from build123d import *

# Parameters (mm, degrees)
SKETCH3_W           = 31.27
SKETCH3_H           = 42.48
BOSS_EXTRUDE1_DEPTH = 6
SKETCH4_R           = 4.7
BOSS_EXTRUDE2_DEPTH = 6
SKETCH6_R           = 5.1
CUT_EXTRUDE2_DEPTH  = 6
FILLET1_R           = 2
FILLET2_R           = 2


with BuildPart() as part:
    # Sketch3 → Boss-Extrude1 (new body)
    with BuildSketch(Plane(origin=(0, 0, 0), x_dir=(1, 0, 0), z_dir=(0, 1, 0))):
        Rectangle(SKETCH3_W, SKETCH3_H)
    extrude(amount=BOSS_EXTRUDE1_DEPTH)

    # Sketch4 → Boss-Extrude2 (add)
    with BuildSketch(Plane(origin=(15.635, 0, 0), x_dir=(0, 0, -1), z_dir=(1, 0, 0))):
        with BuildLine():
            Line((-24.997886253, 0), (25.03656642, 0))
            Line((25.03656642, 0), (25.03656642, 10.942584388))
            Line((25.03656642, 10.942584388), (37.020669589, 23))
            Line((37.020669589, 23), (19.258864986, 40.653807887))
            ThreePointArc((19.258864986, 40.653807887), (-11.905269618, 62.875361443), (-15.817481327, 24.800496669))
            Line((-15.817481327, 24.800496669), (-24.997886253, 12.19))
            Line((-24.997886253, 12.19), (-24.997886253, 0))
        make_face()
        with Locations((-2.786694922, 42.7)):
            Circle(SKETCH4_R, mode=Mode.SUBTRACT)
    boss_extrude2 = extrude(amount=BOSS_EXTRUDE2_DEPTH)

    # Mirror2: Boss-Extrude2 across plane
    add(boss_extrude2.mirror(Plane(origin=(0, 0, 0), x_dir=(0, 0, 1), z_dir=(1, 0, 0))))

    # Sketch6 → Cut-Extrude2 (cut)
    with BuildSketch(Plane.XZ):
        with Locations(Location((0, 0, 0), (0, 0, 270))):
            Circle(SKETCH6_R)
    extrude(amount=-CUT_EXTRUDE2_DEPTH, mode=Mode.SUBTRACT)

    # Fillet1
    fillet1_edges = [part.edges().sort_by_distance(p)[0] for p in [
        (-18.635, 12.19, 24.997886253),
        (-18.635, 0, 24.997886253),
        (18.635, 10.942584388, -25.03656642),
        (-18.635, 10.942584388, -25.03656642),
        (-18.635, 0, -25.03656642),
        (18.635, 0, -25.03656642),
        (18.635, 0, 24.997886253),
        (18.635, 12.19, 24.997886253),
        (18.635, 24.800496669, 15.817481327),
        (-18.635, 24.800496669, 15.817481327),
        (18.635, 23, -37.020669589),
        (-18.635, 23, -37.020669589),
    ]]
    fillet(fillet1_edges, radius=FILLET1_R)

    # Fillet2
    fillet2_edges = [part.edges().sort_by_distance(p)[0] for p in [
        (18.635, 40.653807887, -19.258864986),
        (-18.635, 40.653807887, -19.258864986),
    ]]
    fillet(fillet2_edges, radius=FILLET2_R)


solid = part.part
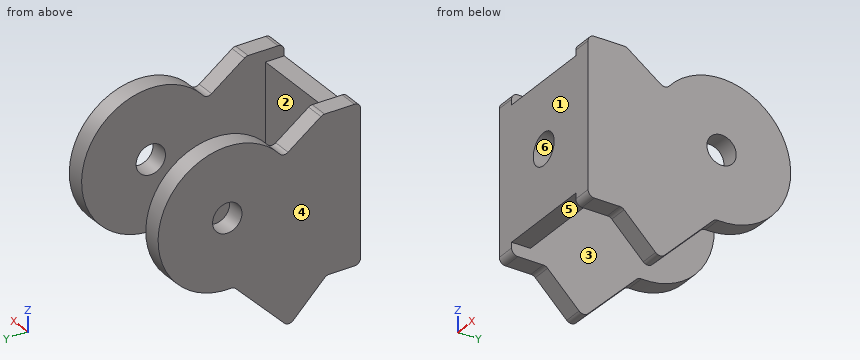
Read the model definition and answer for the solid it produces. Units are mm, in the model's axes. Face numbers are marked on the shaded views. A direction names the side the tool comes from. Round coordinates to 2 decimals unless told otherwise and drop trailing zeros. Write each loop counter-clockwise with the first axis right and the second up, starting at its lowest first coordinate (ties: lowest second). Pieces come first, ordered by that corner, then holes.
1. Straight lines are drawn through the part: L1, parallel to X at y = 3.05, z = 0 (3 decimals); L2, parallel to X at y = 40, z = 22 (3 decimals); L3, parallel to Y at x = -1, z = 5.5. For each, find the intervals that lie inside material, in ascending order.
2. The part is cut by section D-D, the plane z = 6.5. Determine the outline of the cut face in (x, y) (3 decimals), then the cut area to 3 significant figures.
3. Which of the six approach directions +Z, -Z, +X, -X, +Y, -Y give full straight-line access (tool end or side, diameter ignored) to the marked faces 5 and 6?
4. The part is cut by section C-C, the plane y = 7.5. Determine the outline of the cut face in (x, z) (3 decimals), then the cut area to 3 significant figures.
5. The part is cut by section A-A, the plane y = 42.7. Determine the outline of the cut face in (x, z) (3 decimals), then the cut area to 3 significant figures.
6. The part is cut by section B-B, the plane x = 0. Determine the outline of the cut face in (y, z).
7. Given pin 1 Ø10 at (x, z) = (-7, -0.5) entering from +Y; pin 2 Ø6.5 at (x, y) = (18.5, 5) entering from -Z; pin 3 Ø1.8 at (x, y) = (-4, 2.5) entering from +Z; pin 4 Ø3 at (x, y) = (13.5, 46.5) entering from +Z (3 decimals), each flat-ended and moving along its own axis, determine where each tip first touches the part or whether it passes through.
8. Determine the mould class of the marked faces 1, 2, 3 and 4 for opening direction X: pulls with the +X half, pulls with the -X half, needs draft (parallel to the pull), parting line crosses it, or undercut.
Values:
1. L1: x = -21.635 to -5.1, 5.1 to 21.635
1. L2: x = -21.635 to -15.635, 15.635 to 21.635
1. L3: y = 0 to 6
2. outline: (-21.635, 0) - (21.635, 0) - (21.635, 39.819) - (15.635, 39.819) - (15.635, 6) - (-15.635, 6) - (-15.635, 39.819) - (-21.635, 39.819) - close; (-21.635, 45.581) - (-15.635, 45.581) - (-15.635, 64.527) - (-21.635, 64.527) - close; (15.635, 45.581) - (21.635, 45.581) - (21.635, 64.527) - (15.635, 64.527) - close
2. area: 893 mm2
3. face 5: -Z, +Y, -Y
3. face 6: +Y, -Y
4. outline: (-21.635, -25.037) - (-15.635, -25.037) - (-15.635, 24.998) - (-21.635, 24.998) - close; (15.635, -25.037) - (21.635, -25.037) - (21.635, 24.998) - (15.635, 24.998) - close
4. area: 600 mm2
5. outline: (-21.635, -19.354) - (-15.635, -19.354) - (-15.635, -1.913) - (-21.635, -1.913) - close; (-21.635, 7.487) - (-15.635, 7.487) - (-15.635, 24.927) - (-21.635, 24.927) - close; (15.635, -19.354) - (21.635, -19.354) - (21.635, -1.913) - (15.635, -1.913) - close; (15.635, 7.487) - (21.635, 7.487) - (21.635, 24.927) - (15.635, 24.927) - close
5. area: 419 mm2
6. outline: (0, -21.24) - (6, -21.24) - (6, -5.1) - (0, -5.1) - close; (0, 5.1) - (6, 5.1) - (6, 21.24) - (0, 21.24) - close
7. pin 1: stops at y = 6
7. pin 2: stops at z = -25.04
7. pin 3: stops at z = 21.24
7. pin 4: passes through
8. face 1: needs draft
8. face 2: undercut
8. face 3: undercut
8. face 4: pulls with the -X half
